from build123d import *

# Parameters (mm, degrees)
SKETCH_1_R          = 4
EXTRUDE_1_DEPTH     = 39.5
SKETCH_2_R          = 3
EXTRUDE_2_DEPTH     = 1
SKETCH_3_R          = 4
EXTRUDE_3_DEPTH     = 805.5
SKETCH_4_R          = 3
EXTRUDE_4_DEPTH     = 42.5
CUT_EXTRUDE_1_DEPTH = 5
CHAMFER_1_SIZE      = 1.5


with BuildPart() as part:
    # 草图1 → 凸台-拉伸1 (new body)
    with BuildSketch(Plane.XY):
        Circle(SKETCH_1_R)
    extrude(amount=EXTRUDE_1_DEPTH)

    # 草图2 → 凸台-拉伸2 (add)
    with BuildSketch(Plane.XY.offset(39.5)):
        Circle(SKETCH_2_R)
    extrude(amount=EXTRUDE_2_DEPTH)

    # 草图3 → 凸台-拉伸3 (add)
    with BuildSketch(Plane.XY.offset(40.5)):
        Circle(SKETCH_3_R)
    extrude(amount=EXTRUDE_3_DEPTH)

    # 草图4 → 凸台-拉伸4 (add)
    with BuildSketch(Plane.XY.offset(846)):
        Circle(SKETCH_4_R)
    extrude(amount=EXTRUDE_4_DEPTH)

    # 草图7 → 切除-拉伸1 (cut)
    with BuildSketch(Plane(origin=(0, 0, 0), x_dir=(-1, 0, 0), z_dir=(0, 0, -1))):
        Polygon((3, 0), (1.5, -2.598076211), (-1.5, -2.598076211), (-3, 0), (-1.5, 2.598076211), (1.5, 2.598076211), align=None)
    extrude(amount=-CUT_EXTRUDE_1_DEPTH, mode=Mode.SUBTRACT)

    # 倒角1
    chamfer_1_edges = [part.edges().sort_by_distance(p)[0] for p in [
        (-3, 0, 888.5),
    ]]
    chamfer(chamfer_1_edges, length=CHAMFER_1_SIZE)


solid = part.part
The listing builds one solid part. Answer for the finished solid, in the listing's coordinates (mm). Coordinates: 2 decimals unless noted, no trailing zeros. Order: outer loops, then holes, each group sorted by start corner. A loop starts at its lowest first (then second) coordinate and runs counter-clockwise, first axis right, second up.
Q1. Given P1, Ø2, axis at x = -3, y = 1, coming from the +Z side, flat-ended and moving along its own axis, determine where the tip first touches the part or whether it passes through.
Q2. Consider line 1 (Z direction, x = -3.25, y = -1.25); line 2 (X direction, y = -0.75, z = 519); line 3 (Z direction, x = -0.5, y = 1). Determine where each line is inside the solid, lowest interval first.
Q3. A cutting plane is placed at B-B, the plane z = 706.5. Write down the section's boundary in (x, y), and give its area (3 significant figures).
Q4. A cutting plane is placed at A-A, the plane x = 0. Write down the section's boundary in (y, z), and give its area (3 significant figures).
Answers follow:
1. P1: stops at z = 887.84
2. line 1: z = 0 to 39.5, 40.5 to 846
2. line 2: x = -3.93 to 3.93
2. line 3: z = 5 to 888.5
3. outline: circle Ø8 at (0, 0)
3. area: 50.3 mm2
4. outline: (-4, 0) - (-2.6, 0) - (-2.6, 5) - (2.6, 5) - (2.6, 0) - (4, 0) - (4, 39.5) - (3, 39.5) - (3, 40.5) - (4, 40.5) - (4, 846) - (3, 846) - (3, 887) - (1.5, 888.5) - (-1.5, 888.5) - (-3, 887) - (-3, 846) - (-4, 846) - (-4, 40.5) - (-3, 40.5) - (-3, 39.5) - (-4, 39.5) - close
4. area: 6,990 mm2
